Input: part model. Units: mm. Frame: model coordinates. A direction names the side the tool comes from. Coordinates: 2 decimals unless noted, no trailing zeros. Write each loop counter-clockwise with the first axis right and the second up, starting at its lowest first coordinate (ties: lowest second). Pieces come first, ordered by that corner, then holes.
from build123d import *

# Parameters (mm, degrees)
SKETCH_9_R           = 2
CUT_EXTRUDE_12_DEPTH = 20
SKETCH_13_W          = 2
SKETCH_13_H          = 3


with BuildPart() as part:
    # 草图8 → 旋转2 (revolve)
    with BuildSketch(Plane(origin=(0, 0, 0), x_dir=(1, 0, 0), z_dir=(0, 1, 0)), mode=Mode.PRIVATE) as revolve_2_sk:
        Polygon((0, 0), (12, 0), (12, -6), (8, -6), (8, -65), (7, -66), (0, -66), align=None)
    revolve(revolve_2_sk.sketch.rotate(Axis((0, 0, 0), (0, 0, 1)), 180), axis=Axis((0, 0, 0), (0, 0, 1)))

    # 草图9 → 切除-拉伸12 (cut)
    with BuildSketch(Plane(origin=(9, 0, 0), x_dir=(0, 0, -1), z_dir=(1, 0, 0))):
        with Locations((-61, 0)):
            Circle(SKETCH_9_R)
    extrude(amount=-CUT_EXTRUDE_12_DEPTH, mode=Mode.SUBTRACT)

    # 草图13 → 切除-旋转3 (revolve, cut)
    with BuildSketch(Plane(origin=(0, 0, 0), x_dir=(1, 0, 0), z_dir=(0, 1, 0)), mode=Mode.PRIVATE) as cut_revolve_3_sk:
        with Locations((7.5, -57.45)):
            Rectangle(SKETCH_13_W, SKETCH_13_H)
    revolve(cut_revolve_3_sk.sketch.rotate(Axis((0, 0, 0), (0, 0, 1)), 180), axis=Axis((0, 0, 0), (0, 0, 1)), mode=Mode.SUBTRACT)


solid = part.part
Item 1: Pin query (flat end, axial travel): pin 1 Ø5 at (x, y) = (-5.5, 8.5) entering from +Z; pin 2 Ø8 at (y, z) = (1, 13.5) entering from -X; pin 3 Ø6 at (x, z) = (8.5, 36) entering from +Y; pin 4 Ø3.5 at (y, z) = (0, 61) entering from -X. Return the tip coordinate at first contact, or that it passes through.
Item 2: Pull-direction query (Y, two-part tool) for faces 1 (the face through (5.158, 3.955, 57.429)), 2 (the face through (0, 0, 66)), 3 (the face through (0, 0, 63)); classes: released by +Y, released by -Y, zero draft, split by the parting line, or undercut.
Item 3: Section query C-C, the plane z = 61. Return loops of the section in (x, y).
Item 4: Section query B-B, the plane x = 0. Return loops of the section in (y, z), then the cut area to 3 significant figures.
Item 5: Access query for faces 4 (the face through (0, -7, 55.95)), 5 (the face through (-11.446, -3.604, 3.042)), 6 (the face through (-2, 8, 6)). Directions: +Z, -Z, +X, -X, +Y, -Y. A direction counts if a zero-diameter tool reaches every point of the face in a straight line with its end or side. Return the directions, or none.
Item 6: Section query A-A, the plane y = 0. Return loops of the section in (x, z).
Item 7: Section query D-D, the plane z = 34.5. Return loops of the section in (x, y).
Item 8: Material intervals for line 1 (Z direction, x = -4, y = 0); line 2 (Z direction, x = 0.75, y = -9.25); line 3 (Z direction, x = -3.75, y = -1.25), sorted ascending.
The answers:
1. pin 1: stops at z = 65.38
1. pin 2: stops at x = -8
1. pin 3: stops at y = 5.81
1. pin 4: passes through
2. face 1: split by the parting line
2. face 2: zero draft
2. face 3: undercut
3. outline: (-7.75, -2) arc R8 ccw to (7.75, -2) - close; (-7.75, 2) - (7.75, 2) arc R8 ccw to start
4. outline: (-12, 0) - (12, 0) - (12, 6) - (8, 6) - (8, 55.95) - (6.5, 55.95) - (6.5, 58.95) - (8, 58.95) - (8, 65) - (7, 66) - (-7, 66) - (-8, 65) - (-8, 58.95) - (-6.5, 58.95) - (-6.5, 55.95) - (-8, 55.95) - (-8, 6) - (-12, 6) - close; hole circle Ø4 at (0, 61)
4. area: 1,080 mm2
5. face 4: none
5. face 5: +Z, -Z
5. face 6: +Z
6. outline: (-12, 0) - (12, 0) - (12, 6) - (8, 6) - (8, 55.95) - (6.5, 55.95) - (6.5, 58.95) - (8, 58.95) - (8, 59) - (-8, 59) - (-8, 58.95) - (-6.5, 58.95) - (-6.5, 55.95) - (-8, 55.95) - (-8, 6) - (-12, 6) - close; (-8, 63) - (8, 63) - (8, 65) - (7, 66) - (-7, 66) - (-8, 65) - close
7. outline: circle Ø16 at (0, 0)
8. line 1: z = 0 to 59, 63 to 66
8. line 2: z = 0 to 6
8. line 3: z = 0 to 59.44, 62.56 to 66
